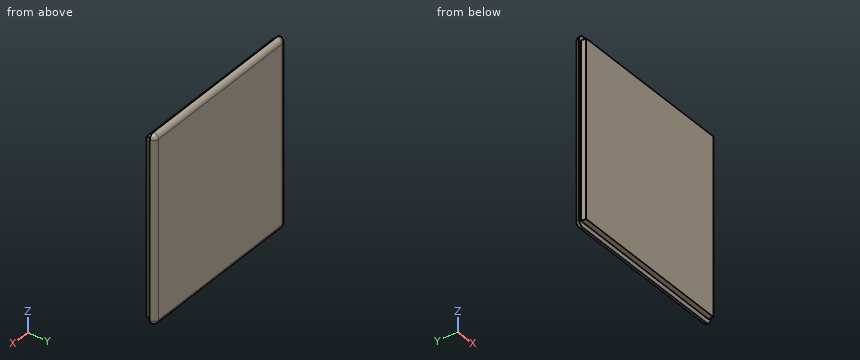
```python
from build123d import *

# Parameters (mm, degrees)
SKETCH_1_W      = 34
SKETCH_1_H      = 35
EXTRUDE_2_DEPTH = 1
SKETCH_3_W      = 35
SKETCH_3_H      = 37
EXTRUDE_3_DEPTH = 1
FILLET_1_R      = 1


with BuildPart() as part:
    # ｽｹｯﾁ1 → ﾎﾞｽ - 押し出し2 (new body)
    with BuildSketch(Plane(origin=(0, 0, 0), x_dir=(1, 0, 0), z_dir=(0, 1, 0))):
        with Locations((0.317073171, 2.724137931)):
            Rectangle(SKETCH_1_W, SKETCH_1_H)
    extrude(amount=EXTRUDE_2_DEPTH)

    # ｽｹｯﾁ3 → ﾎﾞｽ - 押し出し3 (add)
    with BuildSketch(Plane(origin=(0, 1, 0), x_dir=(1, 0, 0), z_dir=(0, 1, 0))):
        with Locations((0.317073171, 2.724137931)):
            Rectangle(SKETCH_3_W, SKETCH_3_H)
    extrude(amount=EXTRUDE_3_DEPTH)

    # ﾌｨﾚｯﾄ1
    fillet_1_edges = [part.edges().sort_by_distance(p)[0] for p in [
        (-17.182926829, 1.5, -21.224137931),
        (-17.182926829, 1.5, 15.775862069),
        (17.817073171, 1.5, 15.775862069),
        (17.817073171, 1.5, -21.224137931),
        (-17.182926829, 2, -2.724137931),
        (0.317073171, 2, 15.775862069),
        (17.817073171, 2, -2.724137931),
        (0.317073171, 2, -21.224137931),
    ]]
    fillet(fillet_1_edges, radius=FILLET_1_R - 0.0001)  # a hair under: the kernel refuses the full size


solid = part.part
```
Part model, mm, in its own coordinate system. Give positions to 0.01 mm unless a question says otherwise; leave off trailing zeros. Order: outer loops, then holes, each group sorted by start corner. A loop starts at its lowest first (then second) coordinate and runs counter-clockwise, first axis right, second up. Notation, with made-up numbers: (15, -39) - (56, -39) arc R31 cw to (56, -12) - close; hole circle Ø4 at (29.25, 30.25). An arc over 180 degrees is marked (long way). Use one line per item in the form item = value.
Item 1: Probe probe 1 along Z at (x, y) = (13, 1.05); probe 2 along Z at (x, y) = (8.5, 0.5); probe 3 along X at (y, z) = (0.95, -16). List the from-to ranges inside material, lowest first. Write a range as from..to.
Solution:
probe_1 = -21.22..15.77
probe_2 = -20.22..14.78
probe_3 = -16.68..17.32
Item 2: Pin check, flat tips, straight feed: pin 1 Ø0.8 at (y, z) = (0.5, 3) entering from -X; pin 2 Ø0.5 at (y, z) = (0.5, 1) entering from +X. Stop position of each tip, or through.
Solution:
pin_1 = -16.68
pin_2 = 17.32
Item 3: Slice it at C-C on y = 1.6. Give the cut face in (x, z), and give its area (3 significant figures).
Solution:
outline = (-16.98, -20.22) arc R0.8 ccw to (-16.18, -21.02) - (16.82, -21.02) arc R0.8 ccw to (17.62, -20.22) - (17.62, 14.78) arc R0.8 ccw to (16.82, 15.58) - (-16.18, 15.58) arc R0.8 ccw to (-16.98, 14.78) - close
area = 1,270 mm2
